```python
from build123d import *

# Parameters (mm, degrees)
SKETCH_1_R      = 2
SKETCH_1_R_2    = 1
SKETCH_1_W      = 10
SKETCH_1_H      = 3
EXTRUDE_1_DEPTH = 3


with BuildPart() as part:
    # 草图1 → 凸台-拉伸1 (new body)
    with BuildSketch(Plane.XY):
        Polygon((-35, 17.5), (-35, 15.5), (-38, 15.5), (-38, 5.5), (-35, 5.5), (-35, -5.5), (-38, -5.5), (-38, -15.5), (-35, -15.5), (-35, -17.5), (-35, -22.5), (35, -22.5), (35, -17.5), (35, -15.5), (38, -15.5), (38, -5.5), (35, -5.5), (35, 5.5), (38, 5.5), (38, 15.5), (35, 15.5), (35, 17.5), (35, 22.5), (-35, 22.5), align=None)
        with Locations((0, 14)):
            Circle(SKETCH_1_R, mode=Mode.SUBTRACT)
        with Locations(Location((0, -14, 0), (0, 0, 180))):
            Circle(SKETCH_1_R, mode=Mode.SUBTRACT)
        with Locations((22, 10)):
            Circle(SKETCH_1_R_2, mode=Mode.SUBTRACT)
        with Locations((22, -10)):
            Circle(SKETCH_1_R_2, mode=Mode.SUBTRACT)
        with Locations((-22, -10)):
            Circle(SKETCH_1_R_2, mode=Mode.SUBTRACT)
        with Locations((-22, 10)):
            Circle(SKETCH_1_R_2, mode=Mode.SUBTRACT)
        with Locations((0, 19)):
            Rectangle(SKETCH_1_W, SKETCH_1_H, mode=Mode.SUBTRACT)
        with Locations((-15, 19)):
            Rectangle(SKETCH_1_W, SKETCH_1_H, mode=Mode.SUBTRACT)
        with Locations((15, 19)):
            Rectangle(SKETCH_1_W, SKETCH_1_H, mode=Mode.SUBTRACT)
        with Locations((15, -19)):
            Rectangle(SKETCH_1_W, SKETCH_1_H, mode=Mode.SUBTRACT)
        with Locations((0, -19)):
            Rectangle(SKETCH_1_W, SKETCH_1_H, mode=Mode.SUBTRACT)
        with Locations((-15, -19)):
            Rectangle(SKETCH_1_W, SKETCH_1_H, mode=Mode.SUBTRACT)
    extrude(amount=EXTRUDE_1_DEPTH)


solid = part.part
```
The listing builds one solid part. Answer for the finished solid, in the listing's coordinates (mm). A direction names the side the tool comes from. Coordinates: 2 decimals unless noted, no trailing zeros. Write each loop counter-clockwise with the first axis right and the second up, starting at its lowest first coordinate (ties: lowest second). Pieces come first, ordered by that corner, then holes. Notation, with made-up numbers: M 71.5,45.25 L 88.5,45.25 A17 ccw 88.5,66.25 Z; hole C 74,-21.75 d9. An arc over 180 degrees is marked long. Use a Markdown table: item, result. Add a question column.
1. Straight lines are drawn through the part: line 1 along X through (y, z) = (-19, 2.55); line 2 along Y through (x, z) = (22, 0.8); line 3 along Y through (x, z) = (14.5, 2.2). For each, find the intervals that lie inside material, in ascending order. Write a range as [from, to].
2. Section C-C (y = 14) is taken. Give the vertices of the cut face in (x, z), plus the area to 3 significant figures.
3. Which of the six approach directions +Z, -Z, +X, -X, +Y, -Y give full straight-line access (tool end or side, diameter ignored) to faces 1 (the flat face through (-35, 19, 1)), 2 (the flat face through (10, 19, 1)), 3 (the flat face through (-37, -15.5, 1))?
4. Section B-B (x = 19) is taken. Give the vertices of the cut face in (y, z), plus the area to 3 significant figures.
5. Section D-D (y = -18.5) is taken. Give the vertices of the cut face in (x, z).
6. For a pull along X with two mould halves and no side action, classify faces 4 (the flat face through (35, -19, 1)), 5 (the flat face through (-38, 11, 1)), 6 (the flat face through (-37, 5.5, 1)), 7 (the cylindrical face through (-22, -9, 1)) as +X half, -X half, draft (parallel to the pull), parting line (faces both ways), or undercut.
7. Given P1, Ø1.5, axis at x = 36.5, z = 2, coming from the -Y side; P2, Ø1, axis at y = -4.5, z = 0.5, coming from the +X side; P3, Ø1.5, axis at y = 19.5, z = 1.5, coming from the -X side, each flat-ended and moving along its own axis, determine where each tip first touches the part or whether it passes through.
8. Section A-A (y = -10) is taken. Give the vertices of the cut face in (x, z), plus the area to 3 significant figures.
Data:
| question | item | result |
|---|---|---|
| 1 | line 1 | x = [-35, -20], [-10, -5], [5, 10], [20, 35] |
| 1 | line 2 | y = [-22.5, -11], [-9, 9], [11, 22.5] |
| 1 | line 3 | y = [-22.5, -20.5], [-17.5, 17.5], [20.5, 22.5] |
| 2 | outline | M -38,0 L -2,0 L -2,3 L -38,3 Z; M 2,0 L 38,0 L 38,3 L 2,3 Z |
| 2 | area | 216 mm2 |
| 3 | face 1 | +Z, -Z, -X, +Y |
| 3 | face 2 | +Z, -Z |
| 3 | face 3 | +Z, -Z, -X, -Y |
| 4 | outline | M -22.5,0 L -20.5,0 L -20.5,3 L -22.5,3 Z; M -17.5,0 L 17.5,0 L 17.5,3 L -17.5,3 Z; M 20.5,0 L 22.5,0 L 22.5,3 L 20.5,3 Z |
| 4 | area | 117 mm2 |
| 5 | outline | M -35,0 L -20,0 L -20,3 L -35,3 Z; M -10,0 L -5,0 L -5,3 L -10,3 Z; M 5,0 L 10,0 L 10,3 L 5,3 Z; M 20,0 L 35,0 L 35,3 L 20,3 Z |
| 6 | face 4 | +X half |
| 6 | face 5 | -X half |
| 6 | face 6 | draft |
| 6 | face 7 | undercut |
| 7 | P1 | stops at y = -15.5 |
| 7 | P2 | stops at x = 35 |
| 7 | P3 | stops at x = -35 |
| 8 | outline | M -38,0 L -23,0 L -23,3 L -38,3 Z; M -21,0 L 21,0 L 21,3 L -21,3 Z; M 23,0 L 38,0 L 38,3 L 23,3 Z |
| 8 | area | 216 mm2 |
